```python
from build123d import *

# Parameters (mm, degrees)
SKETCH1_R           = 76
BOSS_EXTRUDE1_DEPTH = 3.5
CUT_EXTRUDE1_DEPTH  = 4.5
SKETCH3_R           = 1.75
CUT_EXTRUDE2_DEPTH  = 4.5
SKETCH5_R           = 1.25
CUT_EXTRUDE3_DEPTH  = 4.5


with BuildPart() as part:
    # Sketch1 → Boss-Extrude1 (new body)
    with BuildSketch(Plane(origin=(0, 0, 0), x_dir=(1, 0, 0), z_dir=(0, 1, 0))):
        Circle(SKETCH1_R)
    extrude(amount=BOSS_EXTRUDE1_DEPTH)

    # Sketch2 → Cut-Extrude1 (cut, through all)
    with BuildSketch(Plane(origin=(0, 3.5, 0), x_dir=(1, 0, 0), z_dir=(0, 1, 0))):
        with BuildLine():
            Line((-49.893169191, 51.382751627), (-49.893169191, -51.382751627))
            ThreePointArc((-49.893169191, -51.382751627), (-71.620635969, 0), (-49.893169191, 51.382751627))
        make_face()
        with BuildLine():
            Line((-43.644274738, 56.786378466), (-43.644274738, -56.786378466))
            ThreePointArc((-43.644274738, -56.786378466), (0, -71.620635969), (43.644274738, -56.786378466))
            Line((43.644274738, -56.786378466), (43.644274738, 56.786378466))
            ThreePointArc((43.644274738, 56.786378466), (0, 71.620635969), (-43.644274738, 56.786378466))
        make_face()
        with BuildLine():
            Line((49.893169191, 51.382751627), (49.893169191, -51.382751627))
            ThreePointArc((49.893169191, -51.382751627), (71.620635969, 0), (49.893169191, 51.382751627))
        make_face()
    extrude(amount=-CUT_EXTRUDE1_DEPTH, mode=Mode.SUBTRACT)

    # Sketch3 → Cut-Extrude2 (cut, through all)
    with BuildSketch(Plane(origin=(0, 3.5, 0), x_dir=(1, 0, 0), z_dir=(0, 1, 0))):
        with Locations((-46.793169191, 0)):
            Circle(SKETCH3_R)
        with Locations((46.793169191, 0)):
            Circle(SKETCH3_R)
    extrude(amount=-CUT_EXTRUDE2_DEPTH, mode=Mode.SUBTRACT)

    # Sketch5 → Cut-Extrude3 (cut, through all)
    with BuildSketch(Plane(origin=(0, 3.5, 0), x_dir=(1, 0, 0), z_dir=(0, 1, 0))):
        with Locations((0, -73.75)):
            Circle(SKETCH5_R)
        with Locations((-73.75, 0)):
            Circle(SKETCH5_R)
        with Locations((73.75, 0)):
            Circle(SKETCH5_R)
        with Locations((0, 73.75)):
            Circle(SKETCH5_R)
    extrude(amount=-CUT_EXTRUDE3_DEPTH, mode=Mode.SUBTRACT)


solid = part.part
```
The model under review builds one solid part; all positions refer to its coordinate system, in mm. A direction names the side the tool comes from. Round coordinates to 2 decimals unless told otherwise and drop trailing zeros. Write each loop counter-clockwise with the first axis right and the second up, starting at its lowest first coordinate (ties: lowest second). Pieces come first, ordered by that corner, then holes.
(1) We need section D-D on x = -61. Give the boundary of the cut face in (y, z).
(2) Mouldability with a two-part tool opening along X and no side actions: class faces 3 (the cylindrical face through (35.069, 1.726, 67.425)), 4 (the flat face through (-45, 3.5, -6)), 5 (the cylindrical face through (-48.54, 1.77, -0.08)) as +X half, -X half, draft (parallel to the pull), parting line (faces both ways), or undercut.
(3) We need section A-A on x = 13. Give the boundary of the cut face in (y, z), and give its area (3 significant figures).
(4) We need section B-B on z = -29. Give the boundary of the cut face in (x, y), and give its area (3 significant figures).
(5) Insertion check: pin 1 (1.5 mm diameter, centred on x = -5, y = 2.5, fed in from -Z); pin 2 (3 mm diameter, centred on x = 73.75, z = 0, fed in from -Y); pin 3 (1 mm diameter, centred on y = 1, z = 2.5, fed in from +X); pin 4 (1.8 mm diameter, centred on y = 2.5, z = 5.5, fed in from -X). Each pin has a flat end and moves straight along its axis. Give the tip position at first contact, or say it passes through.
(6) Wall thickness on L1, parallel to X at y = 2.65, z = -43.5; L2, parallel to X at y = 1.05, z = -22; L3, parallel to X at y = 1.55, z = 1.5: over which ranges is each line inside the solid? List them lowest first.
(7) We need section C-C on y = 0.75. Give the number of separate pieces and of enclosed holes in the cut face, and give its area (3 significant figures).
(8) Machinability: for faces 1 (the flat face through (-45, 0, -6)), 2 (the flat face through (-49.893, 2, -1)), which of the approach directions +Z, -Z, +X, -X, +Y, -Y give a long, thin tool a straight path to every point of the face, cutting with its end or side? Answer none if there is none.
Findings below:
1. outline: (0, -45.33) - (3.5, -45.33) - (3.5, -37.53) - (0, -37.53) - close; (0, 37.53) - (3.5, 37.53) - (3.5, 45.33) - (0, 45.33) - close
2. face 3: parting line
2. face 4: draft
2. face 5: undercut
3. outline: (0, -74.88) - (3.5, -74.88) - (3.5, -70.43) - (0, -70.43) - close; (0, 70.43) - (3.5, 70.43) - (3.5, 74.88) - (0, 74.88) - close
3. area: 31.1 mm2
4. outline: (-70.25, 0) - (-65.49, 0) - (-65.49, 3.5) - (-70.25, 3.5) - close; (-49.89, 0) - (-43.64, 0) - (-43.64, 3.5) - (-49.89, 3.5) - close; (43.64, 0) - (49.89, 0) - (49.89, 3.5) - (43.64, 3.5) - close; (65.49, 0) - (70.25, 0) - (70.25, 3.5) - (65.49, 3.5) - close
4. area: 77.1 mm2
5. pin 1: stops at z = -75.88
5. pin 2: stops at y = 0
5. pin 3: stops at x = 75.97
5. pin 4: stops at x = -75.86
6. L1: x = -62.32 to -56.9, -49.89 to -43.64, 43.64 to 49.89, 56.9 to 62.32
6. L2: x = -72.75 to -68.16, -49.89 to -43.64, 43.64 to 49.89, 68.16 to 72.75
6. L3: x = -75.99 to -71.6, -49.89 to -47.69, -45.89 to -43.64, 43.64 to 45.89, 47.69 to 49.89, 71.6 to 75.99
7. separate pieces: 1
7. enclosed holes: 9
7. area: 3,350 mm2
8. face 1: +Z, -Z, +X, -X, -Y
8. face 2: +Y, -Y
